```python
from build123d import *

# Parameters (mm, degrees)
SKETCH1_W               = 40
SKETCH1_H               = 40
SKETCH1_R               = 6.25
BOSS_EXTRUDE1_DEPTH     = 20
SKETCH2_R               = 1.7
CUT_EXTRUDE1_DEPTH      = 11
CUT_EXTRUDE2_START      = -7
CUT_EXTRUDE2_DEPTH      = 1.8
CUT_EXTRUDE3_REACH      = 50.99
CUT_EXTRUDE3_END_RADIUS = 6.25
SKETCH4_R               = 1.7
CUT_EXTRUDE4_START      = -8.45
CUT_EXTRUDE4_DEPTH      = 1.8
SKETCH6_R               = 3.5
CUT_EXTRUDE5_DEPTH      = 3.45
FILLET1_R               = 20
CUT_EXTRUDE6_DEPTH      = 35.641016325


with BuildPart() as part:
    # Sketch1 → Boss-Extrude1 (new body)
    with BuildSketch(Plane(origin=(0, 0, 0), x_dir=(1, 0, 0), z_dir=(0, 1, 0))):
        Rectangle(SKETCH1_W, SKETCH1_H)
        with Locations(Location((0, 0, 0), (0, 0, 270))):
            Circle(SKETCH1_R, mode=Mode.SUBTRACT)
    extrude(amount=BOSS_EXTRUDE1_DEPTH)

    # Sketch2 → Cut-Extrude1 (cut)
    with BuildSketch(Plane.ZY.offset(20)):
        with Locations((-5, 15)):
            Circle(SKETCH2_R)
        with Locations((15, 15)):
            Circle(SKETCH2_R)
        with Locations((0, 5)):
            Circle(SKETCH2_R)
    cut_extrude1 = extrude(amount=-CUT_EXTRUDE1_DEPTH, mode=Mode.SUBTRACT)

    # Sketch3 → Cut-Extrude2 (cut)
    with BuildSketch(Plane.ZY.offset(20).offset(CUT_EXTRUDE2_START)):
        Polygon((-7.95, 12.05), (-2.05, 12.05), (-2.05, 17.95), (-2.05, 20), (-7.95, 20), (-7.95, 17.95), align=None)
        Polygon((12.05, 12.05), (17.95, 12.05), (17.95, 17.95), (17.95, 20), (12.05, 20), (12.05, 17.95), align=None)
        Polygon((-2.95, 7.95), (2.95, 7.95), (2.95, 2.05), (2.95, 0), (-2.95, 0), (-2.95, 2.05), align=None)
    cut_extrude2 = extrude(amount=-CUT_EXTRUDE2_DEPTH, mode=Mode.SUBTRACT)

    # Cut-Extrude3: up to this cylinder (the profile starts outside it)
    cut_extrude3_end = Plane(origin=(0, 10, 0), z_dir=(0, -1, 0)) * Cylinder(CUT_EXTRUDE3_END_RADIUS, 115.48, mode=Mode.PRIVATE)
    # Sketch4 → Cut-Extrude3 (cut, up to the surface)
    with BuildSketch(Plane.XY.offset(20), mode=Mode.PRIVATE) as cut_extrude3_sk1:
        with Locations((0, 10)):
            Circle(SKETCH4_R)
    cut_extrude3_tool1 = extrude(cut_extrude3_sk1.sketch, amount=-CUT_EXTRUDE3_REACH, mode=Mode.PRIVATE) - cut_extrude3_end
    cut_extrude3 = cut_extrude3_tool1.solids().sort_by_distance((0, 10, 20))[0]
    add(cut_extrude3, mode=Mode.SUBTRACT)

    # Sketch5 → Cut-Extrude4 (cut)
    with BuildSketch(Plane.XY.offset(20).offset(CUT_EXTRUDE4_START)):
        Polygon((-2.95, 12.95), (-2.95, 20), (2.95, 20), (2.95, 12.95), (2.95, 7.05), (-2.95, 7.05), align=None)
    cut_extrude4 = extrude(amount=-CUT_EXTRUDE4_DEPTH, mode=Mode.SUBTRACT)

    # Sketch6 → Cut-Extrude5 (cut)
    with BuildSketch(Plane.XY.offset(20)):
        with Locations((0, 10)):
            Circle(SKETCH6_R)
    cut_extrude5 = extrude(amount=-CUT_EXTRUDE5_DEPTH, mode=Mode.SUBTRACT)

    # Mirror1: Cut-Extrude1, Cut-Extrude2, Cut-Extrude3, Cut-Extrude4, Cut-Extrude5 across plane
    add(cut_extrude1.mirror(Plane(origin=(0, 0, 0), x_dir=(0.7071067811865476, 0, 0.7071067811865476), z_dir=(-0.7071067811865477, 0, 0.7071067811865475))), mode=Mode.SUBTRACT)
    add(cut_extrude2.mirror(Plane(origin=(0, 0, 0), x_dir=(0.7071067811865476, 0, 0.7071067811865476), z_dir=(-0.7071067811865477, 0, 0.7071067811865475))), mode=Mode.SUBTRACT)
    add(cut_extrude3.mirror(Plane(origin=(0, 0, 0), x_dir=(0.7071067811865476, 0, 0.7071067811865476), z_dir=(-0.7071067811865477, 0, 0.7071067811865475))), mode=Mode.SUBTRACT)
    add(cut_extrude4.mirror(Plane(origin=(0, 0, 0), x_dir=(0.7071067811865476, 0, 0.7071067811865476), z_dir=(-0.7071067811865477, 0, 0.7071067811865475))), mode=Mode.SUBTRACT)
    add(cut_extrude5.mirror(Plane(origin=(0, 0, 0), x_dir=(0.7071067811865476, 0, 0.7071067811865476), z_dir=(-0.7071067811865477, 0, 0.7071067811865475))), mode=Mode.SUBTRACT)

    # Fillet1
    # the kernel refuses this fillet: 20 mm, written as the material it takes off along each edge
    with BuildSketch(Plane(origin=(20, -50, 20), x_dir=(-1, 0, 0), z_dir=(0, 1, 0))) as fillet1_piece_1:
        with BuildLine():
            CenterArc((FILLET1_R, -FILLET1_R), FILLET1_R, 90, 90)
            Line((0, -FILLET1_R), (0, 0))
            Line((0, 0), (FILLET1_R, 0))
        make_face()
    extrude(amount=120, mode=Mode.SUBTRACT)

    # Sketch7 → Cut-Extrude6 (cut, through all)
    with BuildSketch(Plane(origin=(0, 20, 0), x_dir=(1, 0, 0), z_dir=(0, 1, 0))):
        with BuildLine():
            Line((-20, 10), (-20, 20))
            Line((-20, 20), (-10, 20))
            ThreePointArc((-10, 20), (-12.928932188, 12.928932188), (-20, 10))
        make_face()
    extrude(amount=-CUT_EXTRUDE6_DEPTH, mode=Mode.SUBTRACT)


solid = part.part
```
Geometry check sheet. Reference: the model listing, model coordinates, mm. A direction names the side the tool comes from. Give positions to 0.01 mm unless a question says otherwise; leave off trailing zeros. Order: outer loops, then holes, each group sorted by start corner. A loop starts at its lowest first (then second) coordinate and runs counter-clockwise, first axis right, second up.
1. Access from +Z, -Z, +X, -X, +Y, -Y to the whole of each face (thin tool, end or side, straight path). Record for faces 1 (the face through (-16.55, 14.35, 16.57)), 2 (the face through (0, 5, -9)), 3 (the face through (-3.497, 10.154, 18.299)).
2. Section check C-C, the plane z = 15. Enter the section's corners in (x, y), and give its area (3 significant figures).
3. Gauge pin test, flat ends, axial feed: pin 1 Ø1.4 at (x, y) = (-12, 14.5) entering from -Z; pin 2 Ø4.5 at (y, z) = (17.5, 14) entering from +X; pin 3 Ø0.5 at (x, z) = (-5, -12) entering from +Y. Record the tip position at first contact, or that the pin passes through.
4. Section check B-B, the plane x = -5. Enter the section's corners in (y, z).
5. Section check A-A, the plane y = 18.75. Give the number of separate pieces and of enclosed holes in the cut face, and give its area (3 significant figures).
6. Release check for a two-part mould opening along Z. For faces 4 (the face through (5, 10, -20)), 5 (the face through (-0.37, 8.34, 14.08)), 6 (the face through (-10, 10, 20)), 7 (the face through (-12, 4, -2.95)) record: pulls with the +Z half, pulls with the -Z half, needs draft (parallel to the pull), parting line crosses it, or undercut.
7. Thickness scan on L1, parallel to X at y = 17, z = -2; L2, parallel to Y at x = 15, z = -10; L3, parallel to Z at x = 17, y = 12.5. Record the ranges inside material, lowest first.
Values follow:
1. face 1: -X
1. face 2: -Z
1. face 3: +Z
2. outline: (-20, 0) - (13.23, 0) - (13.23, 20) - (-11.2, 20) - (-11.2, 16.7) - (-9, 16.7) - (-9, 13.3) - (-11.2, 13.3) - (-11.2, 12.05) - (-13, 12.05) - (-13, 13.3) - (-20, 13.3) - close; (-20, 16.7) - (-13, 16.7) - (-13, 20) - (-20, 20) - close; hole circle Ø3.4 at (0, 10)
2. area: 610 mm2
3. pin 1: stops at z = -15.07
3. pin 2: stops at x = 16.18
3. pin 3: stops at y = 12.05
4. outline: (0, -20) - (13.3, -20) - (13.3, -13) - (12.05, -13) - (12.05, -11.2) - (13.3, -11.2) - (13.3, -9) - (16.7, -9) - (16.7, -11.2) - (20, -11.2) - (20, -3.75) - (0, -3.75) - close; (0, 3.75) - (20, 3.75) - (20, 20) - (0, 20) - close; (16.7, -20) - (20, -20) - (20, -13) - (16.7, -13) - close
5. separate pieces: 1
5. enclosed holes: 7
5. area: 1,250 mm2
6. face 4: pulls with the -Z half
6. face 5: needs draft
6. face 6: pulls with the +Z half
6. face 7: undercut
7. L1: x = -20 to -5.92, 5.92 to 9.75, 11.55 to 20
7. L2: y = 0 to 13.3, 16.7 to 20
7. L3: z = -20 to -13, -11.2 to -2.45, 2.45 to 10.54
